```python
from build123d import *

# Parameters (mm, degrees)
SKETCH1_W           = 88
SKETCH1_H           = 81
BOSS_EXTRUDE1_DEPTH = 3
SKETCH2_R           = 3
SKETCH2_R_2         = 0.5
REGULATOR_DEPTH     = 3
SKETCH3_R           = 4
SKETCH3_R_2         = 1.5
ARDUIONO_DEPTH      = 3
SKETCH4_R           = 3
SKETCH4_R_2         = 0.5
SKETCH4_W           = 37.754434331
SKETCH4_H           = 4.20099223
RELAY_DEPTH         = 3
SKETCH5_R           = 1.5
CUT_EXTRUDE1_DEPTH  = 60.876957171


with BuildPart() as part:
    # Sketch1 → Boss-Extrude1 (new body)
    with BuildSketch(Plane.XY):
        Rectangle(SKETCH1_W, SKETCH1_H)
    extrude(amount=BOSS_EXTRUDE1_DEPTH)

    # Sketch2 → regulator (add)
    # profile 1 of 4: a face of its own
    with BuildSketch(Plane(origin=(0, 0, 0), x_dir=(-1, 0, 0), z_dir=(0, 0, -1))):
        with Locations((12.422333314, 20.490496054)):
            Circle(SKETCH2_R)
        with Locations((12.422333314, 20.490496054)):
            Circle(SKETCH2_R_2, mode=Mode.SUBTRACT)
    # profile 2 of 4: a face of its own
    with BuildSketch(Plane(origin=(0, 0, 0), x_dir=(-1, 0, 0), z_dir=(0, 0, -1))):
        with Locations((29.922333314, 20.490496054)):
            Circle(SKETCH2_R)
        with Locations((29.922333314, 20.490496054)):
            Circle(SKETCH2_R_2, mode=Mode.SUBTRACT)
    # profile 3 of 4: a face of its own
    with BuildSketch(Plane(origin=(0, 0, 0), x_dir=(-1, 0, 0), z_dir=(0, 0, -1))):
        with Locations((12.422333314, 34.290496054)):
            Circle(SKETCH2_R)
        with Locations((12.422333314, 34.290496054)):
            Circle(SKETCH2_R_2, mode=Mode.SUBTRACT)
    # profile 4 of 4: a face of its own
    with BuildSketch(Plane(origin=(0, 0, 0), x_dir=(-1, 0, 0), z_dir=(0, 0, -1))):
        with Locations((29.922333314, 34.290496054)):
            Circle(SKETCH2_R)
        with Locations((29.922333314, 34.290496054)):
            Circle(SKETCH2_R_2, mode=Mode.SUBTRACT)
    extrude(amount=REGULATOR_DEPTH)

    # Sketch3 → arduiono (add)
    # profile 1 of 2: a face of its own
    with BuildSketch(Plane(origin=(0, 0, 0), x_dir=(-1, 0, 0), z_dir=(0, 0, -1))):
        with Locations((-23, 24.859193612)):
            Circle(SKETCH3_R)
        with Locations((-23, 24.859193612)):
            Circle(SKETCH3_R_2, mode=Mode.SUBTRACT)
    # profile 2 of 2: a face of its own
    with BuildSketch(Plane(origin=(0, 0, 0), x_dir=(-1, 0, 0), z_dir=(0, 0, -1))):
        with Locations((-22.552178991, -17.138418896)):
            Circle(SKETCH3_R)
        with Locations((-22.552178991, -17.138418896)):
            Circle(SKETCH3_R_2, mode=Mode.SUBTRACT)
    extrude(amount=ARDUIONO_DEPTH)

    # Sketch4 → relay (add)
    # profile 1 of 5: a face of its own
    with BuildSketch(Plane(origin=(0, 0, 0), x_dir=(-1, 0, 0), z_dir=(0, 0, -1))):
        with Locations((36.272183711, -20.196025136)):
            Circle(SKETCH4_R)
        with Locations((36.272183711, -20.196025136)):
            Circle(SKETCH4_R_2, mode=Mode.SUBTRACT)
    # profile 2 of 5: a face of its own
    with BuildSketch(Plane(origin=(0, 0, 0), x_dir=(-1, 0, 0), z_dir=(0, 0, -1))):
        with Locations((22.672183711, -20.196025136)):
            Circle(SKETCH4_R)
        with Locations((22.672183711, -20.196025136)):
            Circle(SKETCH4_R_2, mode=Mode.SUBTRACT)
    # profile 3 of 5: a face of its own
    with BuildSketch(Plane(origin=(0, 0, 0), x_dir=(-1, 0, 0), z_dir=(0, 0, -1))):
        with Locations((12.678796965, -19.832402608)):
            Circle(SKETCH4_R)
        with Locations((12.678796965, -19.832402608)):
            Circle(SKETCH4_R_2, mode=Mode.SUBTRACT)
    # profile 4 of 5: a face of its own
    with BuildSketch(Plane(origin=(0, 0, 0), x_dir=(-1, 0, 0), z_dir=(0, 0, -1))):
        with Locations((-0.921203035, -19.832402608)):
            Circle(SKETCH4_R)
        with Locations((-0.921203035, -19.832402608)):
            Circle(SKETCH4_R_2, mode=Mode.SUBTRACT)
    # profile 5 of 5: a face of its own
    with BuildSketch(Plane(origin=(0, 0, 0), x_dir=(-1, 0, 0), z_dir=(0, 0, -1))):
        with Locations((17.631890713, -9.658418225)):
            Rectangle(SKETCH4_W, SKETCH4_H)
    extrude(amount=RELAY_DEPTH)

    # Sketch5 → Cut-Extrude1 (cut, through all)
    with BuildSketch(Plane(origin=(0, 0, 0), x_dir=(-1, 0, 0), z_dir=(0, 0, -1))):
        with Locations((-37.5, 38)):
            Circle(SKETCH5_R)
        with Locations((37.5, 38)):
            Circle(SKETCH5_R)
        with Locations((37.5, -38)):
            Circle(SKETCH5_R)
        with Locations((-37.5, -38)):
            Circle(SKETCH5_R)
    extrude(amount=-CUT_EXTRUDE1_DEPTH, mode=Mode.SUBTRACT)


solid = part.part
```
Read the model definition and answer for the solid it produces. Units are mm, in the model's axes. A direction names the side the tool comes from. Give positions to 0.01 mm unless a question says otherwise; leave off trailing zeros. Write each loop counter-clockwise with the first axis right and the second up, starting at its lowest first coordinate (ties: lowest second). Pieces come first, ordered by that corner, then holes. Notation, with made-up numbers: M 74,-15.5 L 128,-15.5 A31 cw 128,12.5 Z; hole C 33,40.5 d11. An arc over 180 degrees is marked long. Put each result on its own line as item: value. Start each with the question number.
1. Consider line 1 along Y through (x, z) = (-37.5, 0.9); line 2 along Y through (x, z) = (23, -1.8); line 3 along Y through (x, z) = (-28, -1.8). Determine where each line is inside the solid, lowest interval first.
2. For a pull along X with two mould halves and no side action, classify faces 1 (the flat face through (1.245, -10, -1)), 2 (the cylindrical face through (26.996, 25.035, -1.479)), 3 (the flat face through (23, -19, -3)) as released by +X, released by -X, zero draft, split by the parting line, or undercut.
3. The part is cut by section B-B, the plane x = 37.5. Give the vertices of the cut face in (y, z).
4. The part is cut by section A-A, the plane y = -38. Give the vertices of the cut face in (x, z), and give its area (3 significant figures).
5. The part is cut by section C-C, the plane x = -18.5. Give the vertices of the cut face in (y, z), and give its area (3 significant figures).
6. Which of the six approach directions +Z, -Z, +X, -X, +Y, -Y give full straight-line access (tool end or side, diameter ignored) to faces 4 (the flat face through (-17, -11.759, -1)), 5 (the cylindrical face through (-32.784, 21.392, -1.479)), 6 (the flat face through (44, -1, 1))?
7. The part is cut by section D-D, the plane y = -6. Give the vertices of the cut face in (x, z).
8. Each of these flat-tipped pins is pushed along its axis until it touches: pin 1 Ø1.5 at (x, y) = (-6, -14.5) entering from -Z; pin 2 Ø2.5 at (x, y) = (37.5, -38) entering from -Z; pin 3 Ø3.5 at (x, z) = (-22.5, -2) entering from +Y. Where does it stop, or does it pass through?
Final values:
1. line 1: y = -40.5 to -39.5, -36.5 to 36.5, 39.5 to 40.5
1. line 2: y = -21.11 to -18.57, -15.71 to -13.16, 20.86 to 23.36, 26.36 to 28.86
1. line 3: y = -11.76 to -7.56, 18.19 to 22.79, 31.99 to 36.59
2. face 1: released by +X
2. face 2: undercut
2. face 3: zero draft
3. outline: M -40.5,0 L -39.5,0 L -39.5,3 L -40.5,3 Z; M -36.5,0 L 36.5,0 L 36.5,3 L -36.5,3 Z; M 39.5,0 L 40.5,0 L 40.5,3 L 39.5,3 Z
4. outline: M -44,0 L -39,0 L -39,3 L -44,3 Z; M -36,0 L 36,0 L 36,3 L -36,3 Z; M 39,0 L 44,0 L 44,3 L 39,3 Z
4. area: 246 mm²
5. outline: M -40.5,0 L -11.76,0 L -11.76,-3 L -7.56,-3 L -7.56,0 L 40.5,0 L 40.5,3 L -40.5,3 Z
5. area: 256 mm²
6. face 4: -Z, +X, -X
6. face 5: -Z
6. face 6: +Z, -Z, +X, +Y, -Y
7. outline: M -44,0 L 44,0 L 44,3 L -44,3 Z
8. pin 1: stops at z = 0
8. pin 2: passes through
8. pin 3: stops at y = -7.56
